Geometry check sheet. Reference: the model listing, model coordinates, mm. A direction names the side the tool comes from. Give positions to 0.01 mm unless a question says otherwise; leave off trailing zeros. Loops run counter-clockwise (first coordinate to the right, second up) from the corner with the lowest first, then second, coordinate; pieces in that order, holes last. Notation, with made-up numbers: (-20, -11) -> (37, -11) arc R31 cw to (37, 18) -> close; hole circle Ø5 at (78, 40.5). An arc over 180 degrees is marked (long way). Write item = value, one per line. Start each with the question number.
```python
from build123d import *

# Parameters (mm, degrees)
BOSS_EXTRUDE1_DEPTH = 14
SKETCH2_R           = 1.25
CUT_EXTRUDE1_DEPTH  = 43
BOSS_EXTRUDE2_DEPTH = 1.5


with BuildPart() as part:
    # Sketch1 → Boss-Extrude1 (new body)
    with BuildSketch(Plane(origin=(0, 0, 0), x_dir=(1, 0, 0), z_dir=(0, 1, 0))):
        Polygon((-19, 1), (19, 1), (19, 8), (21, 8), (21, 1), (21, -1), (21, -8), (19, -8), (19, -1), (-19, -1), (-19, -8), (-21, -8), (-21, -1), (-21, 1), (-21, 8), (-19, 8), align=None)
    extrude(amount=BOSS_EXTRUDE1_DEPTH)

    # Sketch2 → Cut-Extrude1 (cut, through all)
    with BuildSketch(Plane(origin=(21, 0, 0), x_dir=(0, 0, -1), z_dir=(1, 0, 0))):
        with Locations((5, 10)):
            Circle(SKETCH2_R)
        with Locations((5, 4)):
            Circle(SKETCH2_R)
        with Locations((-5, 4)):
            Circle(SKETCH2_R)
        with Locations((-5, 10)):
            Circle(SKETCH2_R)
    extrude(amount=-CUT_EXTRUDE1_DEPTH, mode=Mode.SUBTRACT)

    # Sketch3 → Boss-Extrude2 (add)
    with BuildSketch(Plane(origin=(0, 14, 0), x_dir=(1, 0, 0), z_dir=(0, 1, 0))):
        Polygon((-19, 1), (-19, 6), (-16.5, 3.5), (16.5, 3.5), (19, 6), (19, 1), (14, 1), (-14, 1), align=None)
        Polygon((19, -1), (14, -1), (-14, -1), (-19, -1), (-19, -6), (-16.5, -3.5), (16.5, -3.5), (19, -6), align=None)
    boss_extrude2 = extrude(amount=-BOSS_EXTRUDE2_DEPTH)

    # Mirror1: Boss-Extrude2 across plane
    add(boss_extrude2.mirror(Plane.ZX.offset(7)))


solid = part.part
```
1) Depth check by flat-ended pin: pin 1 Ø5.5 at (x, y) = (-1, 5) entering from -Z; pin 2 Ø3 at (x, y) = (-0.5, 8.5) entering from +Z; pin 3 Ø0.8 at (x, y) = (8, 13) entering from -Z. Enter the tip coordinate at first touch or a pass-through.
2) Section check B-B (z = 5). Give the number of separate pieces and of enclosed holes in the cut face, plus the area to 3 significant figures.
3) Section check C-C (x = 15.5). Enter the section's corners in (y, z), plus the area to 3 significant figures.
4) Tool access check on faces 1 (the flat face through (18, 1, 5)), 2 (the flat face through (-18, 13, -5)), 3 (the flat face through (-19, 7, -5)). Record the directions out of +Z, -Z, +X, -X, +Y, -Y that give a thin tool (end or side, any length) a straight path to the whole face; none if there is none.
5) Section check D-D (z = 2.25). Enter the section's corners in (x, y), plus the area to 3 significant figures.
6) Thickness scan on line 1 (Y direction, x = -20.15, z = -5); line 2 (Y direction, x = -3, z = 1.25); line 3 (X direction, y = 7.75, z = -6.75). Record the ranges inside material, lowest first.
7) Draft check along Z on faces 4 (the flat face through (-18, 1, -5)), 5 (the flat face through (18, 13, 5)), 6 (the cylindrical face through (20.01, 11.24, -4.84)). Enter one of: released by +Z, released by -Z, zero draft, split by the parting line, or undercut.
8) Section check A-A (y = 3.25). Enter the section's corners in (x, z).
Check result:
q1.pin_1 = -1
q1.pin_2 = 1
q1.pin_3 = -3.5
q2.separate_pieces = 6
q2.enclosed_holes = 0
q2.area = 42.0 mm2
q3.outline = (0, -3.5) -> (1.5, -3.5) -> (1.5, -1) -> (12.5, -1) -> (12.5, -3.5) -> (14, -3.5) -> (14, 3.5) -> (12.5, 3.5) -> (12.5, 1) -> (1.5, 1) -> (1.5, 3.5) -> (0, 3.5) -> close
q3.area = 43.0 mm2
q4.face_1 = +Z, +Y, -Y
q4.face_2 = -Z, +Y, -Y
q4.face_3 = -Z
q5.outline = (-21, 0) -> (21, 0) -> (21, 14) -> (-21, 14) -> close; hole (-19, 1.5) -> (19, 1.5) -> (19, 12.5) -> (-19, 12.5) -> close
q5.area = 170 mm2
q6.line_1 = 0 to 2.75, 5.25 to 8.75, 11.25 to 14
q6.line_2 = 0 to 1.5, 12.5 to 14
q6.line_3 = -21 to -19, 19 to 21
q7.face_4 = released by -Z
q7.face_5 = released by +Z
q7.face_6 = undercut
q8.outline = (-21, -8) -> (-19, -8) -> (-19, -6) -> (-21, -6) -> close; (-21, -4) -> (-19, -4) -> (-19, -1) -> (19, -1) -> (19, -4) -> (21, -4) -> (21, 4) -> (19, 4) -> (19, 1) -> (-19, 1) -> (-19, 4) -> (-21, 4) -> close; (-21, 6) -> (-19, 6) -> (-19, 8) -> (-21, 8) -> close; (19, -8) -> (21, -8) -> (21, -6) -> (19, -6) -> close; (19, 6) -> (21, 6) -> (21, 8) -> (19, 8) -> close
